Can you work these out from the model? Positions are in its coordinate system, mm. A direction names the side the tool comes from. Coordinates: 2 decimals unless noted, no trailing zeros. Order: outer loops, then holes, each group sorted by start corner. A loop starts at its lowest first (then second) coordinate and runs counter-clockwise, first axis right, second up. Notation, with made-up numbers: (79.5, -37) -> (119.5, -37) arc R24 cw to (119.5, -24) -> close; hole circle Ø9 at (77, 72). An arc over 180 degrees is marked (long way). Answer as CSV lines item,"result".
from build123d import *

# Parameters (mm, degrees)
SKETCH1_R               = 25
BOSS_EXTRUDE1_DEPTH     = 8
SKETCH2_R               = 4
BOSS_EXTRUDE2_DEPTH     = 15
BOSS_EXTRUDE3_START     = 30
SKETCH3_R               = 4
BOSS_EXTRUDE3_DEPTH     = 30
CUT_EXTRUDE1_DEPTH      = 64.710281745
CUT_EXTRUDE1_DEPTH_BACK = 64.710281745
SKETCH4_R               = 2.5
SKETCH5_R               = 6
BOSS_EXTRUDE4_DEPTH     = 4
BOSS_EXTRUDE5_START     = 4
SKETCH6_R               = 6
BOSS_EXTRUDE5_DEPTH     = 4


with BuildPart() as part:
    # Sketch1 → Boss-Extrude1 (new body)
    with BuildSketch(Plane(origin=(0, 0, 0), x_dir=(1, 0, 0), z_dir=(0, 1, 0))):
        with Locations(Location((0, 0, 0), (0, 0, 270))):
            Circle(SKETCH1_R)
    extrude(amount=BOSS_EXTRUDE1_DEPTH)

    # Sketch2 → Boss-Extrude2 (add)
    with BuildSketch(Plane(origin=(0, 8, 0), x_dir=(1, 0, 0), z_dir=(0, 1, 0))):
        with Locations(Location((0, 0, 0), (0, 0, 270))):
            Circle(SKETCH2_R)
    extrude(amount=BOSS_EXTRUDE2_DEPTH)

    # Sketch3 → Boss-Extrude3 (add)
    with BuildSketch(Plane.XZ.offset(BOSS_EXTRUDE3_START)):
        with Locations(Location((0, 0, 0), (0, 0, 90))):
            Circle(SKETCH3_R)
    extrude(amount=-BOSS_EXTRUDE3_DEPTH)

    # Sketch4 → Cut-Extrude1 (cut, two sides: drawn at the far end of the back side and taken through both)
    with BuildSketch(Plane(origin=(0, 23, 0), x_dir=(1, 0, 0), z_dir=(0, 1, 0)).offset(-CUT_EXTRUDE1_DEPTH_BACK)):
        with Locations(Location((0, 0, 0), (0, 0, 270))):
            Circle(SKETCH4_R)
    extrude(amount=CUT_EXTRUDE1_DEPTH + CUT_EXTRUDE1_DEPTH_BACK, mode=Mode.SUBTRACT)

    # Sketch5 → Boss-Extrude4 (add)
    with BuildSketch(Plane.XZ):
        with Locations(Location((0, 0, 0), (0, 0, 90))):
            Circle(SKETCH5_R)
    extrude(amount=BOSS_EXTRUDE4_DEPTH)

    # Sketch6 → Boss-Extrude5 (add)
    with BuildSketch(Plane(origin=(0, 8, 0), x_dir=(1, 0, 0), z_dir=(0, 1, 0)).offset(BOSS_EXTRUDE5_START)):
        with Locations(Location((0, 0, 0), (0, 0, 270))):
            Circle(SKETCH6_R)
    extrude(amount=-BOSS_EXTRUDE5_DEPTH)


solid = part.part
Q1. Imagine slicing it at D-D (y = -2). List the corners of the cut face in (x, z) for me.
Solution:
outline,"circle Ø12 at (0, 0)"
Q2. For P1, Ø10, axis at x = 3, y = -15, coming from the -Z side; P2, Ø2.5, axis at x = 0, z = -1, coming from the +Y side; P3, Ø2, axis at x = -17, y = 6.5, coming from the -Z side, each with a flat end and sliding along its axis, tell me the tip position at first contact or that it passes through.
Solution:
P1,"z = -4"
P2,"y = 12"
P3,"z = -19.21"
Q3. We'd pull the mould along X, two halves only. Please class faces 1 (the flat face through (-3.92, 12, -1.42)), 2 (the cylindrical face through (-2.44, -17.18, -0.54)), 3 (the cylindrical face through (-2.44, 17.42, -0.54)), 4 (the cylindrical face through (-1.802, -1.972, 5.723)): pulls with the +X half, pulls with the -X half, needs draft (parallel to the pull), parting line crosses it, or undercut.
Solution:
face 1,"needs draft"
face 2,"undercut"
face 3,"undercut"
face 4,"parting line crosses it"
Q4. Which directions (+Z, -Z, +X, -X, +Y, -Y) give clear straight access to the entire face, cutting with the end or side of a thin tool? Please do faces 5 (the cylindrical face through (7.509, 3.944, 23.846)), 6 (the flat face through (0, 8, 0)), 7 (the cylindrical face through (3.905, -17.182, -0.867)), 8 (the flat face through (-5, 8, 5)), 9 (the flat face through (-2, -30, 2)).
Solution:
face 5,"+Y, -Y"
face 6,"none"
face 7,"-Y"
face 8,"+Y"
face 9,"+Z, -Z, +X, -X, -Y"
Q5. Imagine slicing it at C-C (y = -21.5). List the corners of the cut face in (x, z) for me, and give its area (3 significant figures).
Solution:
outline,"circle Ø8 at (0, 0); hole circle Ø5 at (0, 0)"
area,"30.6 mm2"
Q6. If I drill on line 1 (Z direction, x = 0, y = 17.25); line 2 (Y direction, x = -21, z = -10.5), over which ranges is the centre line in solid material (lowest first)?
Solution:
line 1,"-4 to -2.5, 2.5 to 4"
line 2,"0 to 8"
